Part print with two shaded views. Sizes in mm from the minimum x, y, z corner. Coordinates: 2 decimals unless noted, no trailing zeros. Loops run counter-clockwise (first coordinate to the right, second up) from the corner with the lowest first, then second, coordinate; pieces in that order, holes last. Notation, with made-up numbers: (-7, 78) -> (9, 78) arc R14 ccw to (9, 82) -> close; hole circle Ø5 at (84, -36). An arc over 180 degrees is marked (long way). One line per item, written item: value. Start each with the question number.
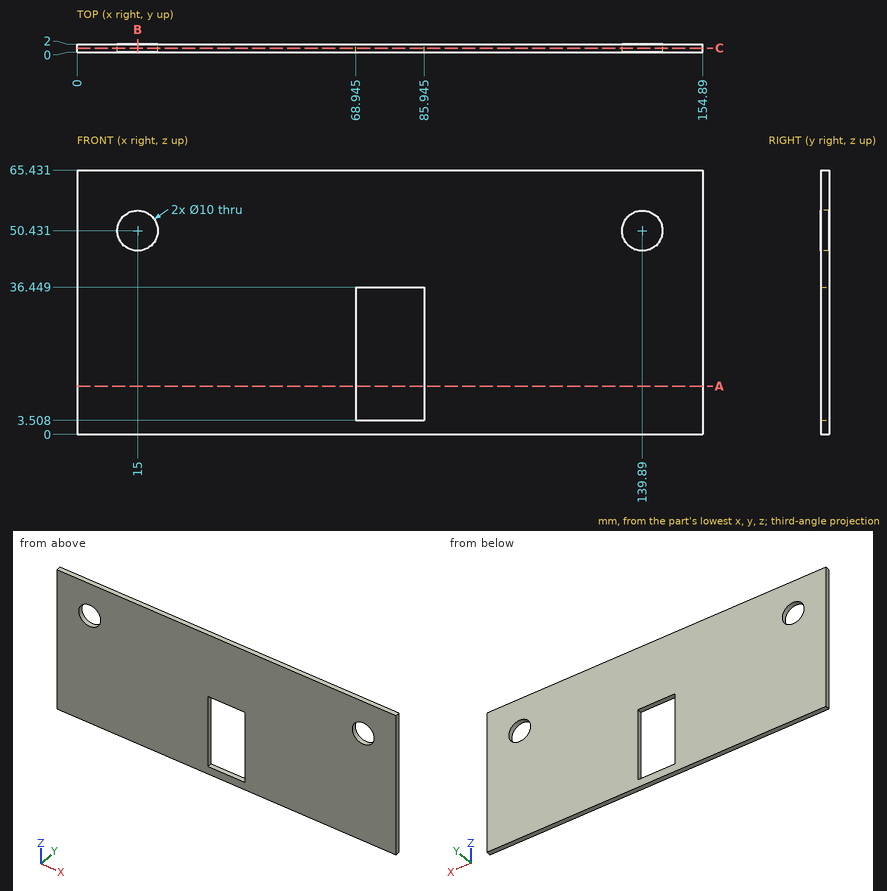
Item 1: Band-saw the part on A-A, the plane z = 12. List the corners of the cut face in (x, y) (1 decimal), and give its area (3 significant figures).
Item 2: Probe probe 1 along Z at (x, y) = (70.5, 1.2); probe 2 along X at (y, z) = (1.2, 35.5) (1 decimal); probe 3 along Z at (x, y) = (140, 0.4). List the from-to ranges inside material, lowest first.
Item 3: Drop a flat-ended pin along its axis: pin 1 Ø8 at (x, z) = (15, 50.43) entering from +Y. Give the stop position or say it passes through.
Item 4: Band-saw the part on C-C, the plane y = 0.95. Count the separate pieces of the cut face and the enclosed holes in it, and give its area (3 significant figures).
Item 5: Band-saw the part on B-B, the plane x = 15. List the corners of the cut face in (y, z).
Worked out:
1. outline: (0, 0) -> (68.9, 0) -> (68.9, 2) -> (0, 2) -> close; (85.9, 0) -> (154.9, 0) -> (154.9, 2) -> (85.9, 2) -> close
1. area: 276 mm²
2. probe 1: z = 0 to 3.51, 36.45 to 65.43
2. probe 2: x = 0 to 68.9, 85.9 to 154.9
2. probe 3: z = 0 to 45.43, 55.43 to 65.43
3. pin 1: passes through
4. separate pieces: 1
4. enclosed holes: 3
4. area: 9,420 mm²
5. outline: (0, 0) -> (2, 0) -> (2, 45.43) -> (0, 45.43) -> close; (0, 55.43) -> (2, 55.43) -> (2, 65.43) -> (0, 65.43) -> close
